Build history of the part. All positions in model axes, mm. A direction names the side the tool comes from. Round coordinates to 2 decimals unless told otherwise and drop trailing zeros. Order: outer loops, then holes, each group sorted by start corner. A loop starts at its lowest first (then second) coordinate and runs counter-clockwise, first axis right, second up. Notation, with made-up numbers: M -40,50.25 L -21,50.25 A13 cw -21,74.25 Z; hole C -6.75,39 d4. An arc over 180 degrees is marked long. One line per item, written item: value. Start each with the question number.
Item 1: Tool access for faces 5 (the flat face through (-1.3, -1.4, 10)), 6 (the cylindrical face through (14.792, -0.014, -0.565)), 7 (the cylindrical face through (-1.708, -0.014, -0.565)): list every direction of +Z, -Z, +X, -X, +Y, -Y with a clear straight run to the whole face (end or side of a thin tool).
Item 2: Two-plate mould, pull along Y, no slides. Class faces 1 (the cylindrical face through (0.014, -1.708, -0.565)), 2 (the cylindrical face through (8.344, 0.715, -0.699)), 3 (the cylindrical face through (1.708, -0.014, -0.565)), 4 (the cylindrical face through (0.014, 1.708, -0.565)): +Y half, -Y half, draft (parallel to the pull), parting line (faces both ways), or undercut.
Item 3: Pin check, flat tips, straight feed: pin 1 (2 mm diameter, centred on x = 4.5, z = 9, fed in from -Y); pin 2 (2 mm diameter, centred on x = -9, z = 8.5, fed in from +Y); pin 3 (1.5 mm diameter, centred on x = 11.5, y = 6, fed in from +Z). Stop position of each tip, or through.
Item 4: Band-saw the part on A-A, the plane z = 8.5. Write the cut outline in (x, y), then the cut area to 3 significant figures.
Item 5: Probe L1, parallel to Y at x = 0, z = 4; L2, parallel to Z at x = 1.5, y = -8; L3, parallel to X at y = -2, z = 11.5. List the from-to ranges inside material, lowest first.
```python
from build123d import *

# Parameters (mm, degrees)
F0_R     = 15
F1_DEPTH = 3
F1_TAPER = 30
F2_DEPTH = 10
F4_DEPTH = 3
F5_R     = 1.5
F6_DEPTH = 10.001
F7_W     = 13.4332590942
F7_H     = 2
F7_W_2   = 2
F7_H_2   = 13.4332590942
F8_DEPTH = 1
F9_R     = 0.99999
F10_R    = 5


# Not quite as in the source:
# - a fillet or chamfer is up to 0.001 mm smaller than in the source, because OpenCascade refuses the exact size


with BuildPart() as f1:
    # F0 (on Top) → F1 (new body)
    with BuildSketch(Plane.XY):
        Circle(F0_R)
    extrude(amount=F1_DEPTH, taper=F1_TAPER)

    # F2 (add): a face of the model
    f2_faces = [f1.faces().sort_by_distance(p)[0] for p in [
        (0, 0, 3),
    ]]
    extrude(f2_faces, amount=F2_DEPTH)

    # F3 (on face) → F4 (cut)
    with BuildSketch(Plane.XY.offset(13)):
        Polygon((2.8, -1.6165807537), (2.8, 1.6165807537), (0, 3.2331615075), (-2.8, 1.6165807537), (-2.8, -1.6165807537), (0, -3.2331615075), align=None)
    extrude(amount=-F4_DEPTH, mode=Mode.SUBTRACT)

    # F5 (on face) → F6 (cut, through all)
    with BuildSketch(Plane.XY.offset(10)):
        Circle(F5_R)
    extrude(amount=-F6_DEPTH, mode=Mode.SUBTRACT)

    # F7 (on face) → F8 (join)
    with BuildSketch(Plane(origin=(0, 0, 0), x_dir=(1, 0, 0), z_dir=(0, 0, -1))):
        with Locations((-8.25, 0)):
            Rectangle(F7_W, F7_H)
        with Locations((0, 8.25)):
            Rectangle(F7_W_2, F7_H_2)
        with Locations((8.25, 0)):
            Rectangle(F7_W, F7_H)
        with Locations((0, -8.25)):
            Rectangle(F7_W_2, F7_H_2)
    extrude(amount=F8_DEPTH)

    # F9 (radius 1 in the source; OpenCascade refuses exactly that, so slightly less here)
    f9_edges = [f1.edges().sort_by_distance(p)[0] for p in [
        (-1, 8.25, -1),
        (1, 8.25, -1),
        (8.25, 1, -1),
        (14.96663, 0, -1),
        (8.25, -1, -1),
        (1.53337, 0, -1),
        (-8.25, 1, -1),
        (-8.25, -1, -1),
        (1, -8.25, -1),
        (-1, -8.25, -1),
        (0, 14.96663, -1),
        (0, 1.53337, -1),
        (0, -1.53337, -1),
        (-1.53337, 0, -1),
        (-14.96663, 0, -1),
        (0, -14.96663, -1),
    ]]
    fillet(f9_edges, radius=F9_R)

    # F10
    f10_edges = [f1.edges().sort_by_distance(p)[0] for p in [
        (-13.267949, 0, 13),
    ]]
    fillet(f10_edges, radius=F10_R)


solid = f1.part
```
Output:
1. face 5: +Z
1. face 6: -Z, +X, +Y, -Y
1. face 7: -Z, +Y, -Y
2. face 1: undercut
2. face 2: +Y half
2. face 3: draft
2. face 4: undercut
3. pin 1: stops at y = -12.74
3. pin 2: stops at y = 10.56
3. pin 3: stops at z = 11.06
4. outline: C 0,0 d26.49; hole C 0,0 d3
4. area: 544 mm²
5. L1: y = -13.27 to -1.5, 1.5 to 13.27
5. L2: z = 0 to 13
5. L3: x = -11.67 to -2.14, 2.14 to 11.67
